from build123d import *

# Parameters (mm, degrees)
F1_DEPTH      = 4.76
F1_DEPTH_BACK = 4.76
F2_R          = 9
F3_DEPTH      = 7.94
F3_DEPTH_BACK = 7.94
F4_R          = 5.55625
F5_DEPTH      = 15.881
F6_R          = 2
F7_DEPTH      = 33.001


with BuildPart() as f1:
    # F0 (on Right) → F1 (new body, two sides)
    with BuildSketch(Plane.YZ) as f1_sk:
        with BuildLine():
            Line((-7.348469, 30), (-13.5, 30))
            Line((-13.5, 30), (-13.5, 3.125))
            Line((-13.5, 3.125), (-22.5, 3.125))
            Line((-22.5, 3.125), (-22.5, 0))
            Line((-22.5, 0), (22.5, 0))
            Line((22.5, 0), (22.5, 3.125))
            Line((22.5, 3.125), (13.5, 3.125))
            Line((13.5, 3.125), (13.5, 30))
            Line((13.5, 30), (7.348469, 30))
            ThreePointArc((7.348469, 30), (0, 33), (-7.348469, 30))
        make_face()
    extrude(amount=F1_DEPTH)
    extrude(f1_sk.sketch, amount=-F1_DEPTH_BACK)

    # F2 (on Right) → F3 (join, two sides)
    with BuildSketch(Plane.YZ) as f3_sk:
        with Locations((0, 22.5)):
            Circle(F2_R)
    extrude(amount=F3_DEPTH)
    extrude(f3_sk.sketch, amount=-F3_DEPTH_BACK)

    # F4 (on face) → F5 (cut, through all)
    with BuildSketch(Plane.YZ.offset(7.94)):
        with Locations((0, 22.5)):
            Circle(F4_R)
    extrude(amount=-F5_DEPTH, mode=Mode.SUBTRACT)

    # F6 (on face) → F7 (cut, through all)
    with BuildSketch(Plane(origin=(0, 0, 0), x_dir=(1, 0, 0), z_dir=(0, 0, -1))):
        with Locations((0, 19.05)):
            Circle(F6_R)
        with Locations((0, -19.05)):
            Circle(F6_R)
    extrude(amount=-F7_DEPTH, mode=Mode.SUBTRACT)


solid = f1.part
Input: part model. Units: mm. Frame: model coordinates. A direction names the side the tool comes from. Give positions to 0.01 mm unless a question says otherwise; leave off trailing zeros. Write each loop counter-clockwise with the first axis right and the second up, starting at its lowest first coordinate (ties: lowest second). Pieces come first, ordered by that corner, then holes.
Q1. Pull-direction query (Y, two-part tool) for faces 4 (the face through (0.11, 2.56, 17.57)), 5 (the face through (-6.328, -1.172, 31.423)), 6 (the face through (1, 17, 3.125)); classes: pulls with the +Y half, pulls with the -Y half, needs draft (parallel to the pull), parting line crosses it, or undercut.
Q2. Section B-B, the plane y = 19.05. Output: boundary loops of the cut face in (x, z) (3 decimals), plus the area to 4 significant figures.
Q3. Section D-D, the plane x = 2.5. Output: boundary loops of the cut face in (y, z) (1 decimal).
Q4. Section A-A, the plane x = 0. State how many separate pieces and enclosed holes the cut face has, plus the area to 3 significant figures.
Q5. Section C-C, the plane z = 22.5. Output: boundary loops of the cut face in (x, y).
Q6. Set-up query: faces 1 (the face through (0, 10, 30)), 2 (the face through (6.328, -1.172, 31.423)), 3 (the face through (0.1, -16.9, 3.125)). Return all of +Z, -Z, +X, -X, +Y, -Y with unobstructed straight access to the full face (end or side cutting, diameter ignored); none if empty.
Q7. First-contact query: P1, Ø3, axis at x = 2.5, z = 12, coming from the +Y side; P2, Ø4.5, axis at x = 0, y = -19.05, coming from the +Z side (3 decimals); P3, Ø1.5, axis at x = -0.5, z = 19, coming from the -Y side. Flat tips, straight axial feed; report the tip coordinate or a pass-through.
Q8. Material intervals for probe 1 along Y at (x, z) = (0, 1.2); probe 2 along Z at (x, y) = (-1.25, 0); probe 3 along X at (y, z) = (19.05, 2.5), sorted ascending.
Filled in:
1. face 4: undercut
1. face 5: parting line crosses it
1. face 6: needs draft
2. outline: (-4.76, 0) - (-2, 0) - (-2, 3.125) - (-4.76, 3.125) - close; (2, 0) - (4.76, 0) - (4.76, 3.125) - (2, 3.125) - close
2. area: 17.25 mm2
3. outline: (-22.5, 0) - (22.5, 0) - (22.5, 3.1) - (13.5, 3.1) - (13.5, 30) - (7.3, 30) arc R10.5 ccw to (-7.3, 30) - (-13.5, 30) - (-13.5, 3.1) - (-22.5, 3.1) - close; hole circle Ø11.1 at (0, 22.5)
4. separate pieces: 3
4. enclosed holes: 1
4. area: 775 mm2
5. outline: (-7.94, -9) - (-4.76, -9) - (-4.76, -13.5) - (4.76, -13.5) - (4.76, -9) - (7.94, -9) - (7.94, -5.56) - (-7.94, -5.56) - close; (-7.94, 5.56) - (7.94, 5.56) - (7.94, 9) - (4.76, 9) - (4.76, 13.5) - (-4.76, 13.5) - (-4.76, 9) - (-7.94, 9) - close
6. face 1: +Z, +X, -X, +Y
6. face 2: +X
6. face 3: +Z, +X, -X, -Y
7. P1: stops at y = 13.5
7. P2: stops at z = 3.125
7. P3: stops at y = -13.5
8. probe 1: y = -22.5 to -21.05, -17.05 to 17.05, 21.05 to 22.5
8. probe 2: z = 0 to 16.94, 28.06 to 33
8. probe 3: x = -4.76 to -2, 2 to 4.76
